Autodesk Inventor part; units mm, degrees
ref_plane "YZ Plane" through (0, 0, 0) normal (1, 0, 0) x (0, 1, 0)
ref_plane "XZ Plane" through (0, 0, 0) normal (0, 1, 0) x (-1, 0, 0)
ref_plane "XY Plane" through (0, 0, 0) normal (0, 0, 1) x (1, 0, 0)
sketch "Sketch1" plane through (0, 0, 0) normal (0, 0, 1) x (1, 0, 0)
  point P0 (0, 0)
sketch "Sketch2" plane through (0, 0, 0) normal (0, 0, 1) x (1, 0, 0)
  circle A0 centre (0, 0) radius 10
  line L0 (2.4793, 73.9585) -> (2.4781, 9.6881)
  line L1 (-2.5359, 9.6731) -> (-2.5218, 9.6731)
  line L2 (-2.5218, 9.6768) -> (-2.5207, 73.9571)
  line L3 (-2.4922, 73.958) -> (2.4781, 9.6881) construction
  line L4 (2.4804, 74.3269) -> (-2.5218, 9.6731) construction
  line L5 (-2.5218, 9.6731) -> (-2.5218, 9.6723)
  line L6 (9.283, 2.5) -> (74.717, 2.5)
  line L7 (74.717, 2.5) -> (74.717, -2.5)
  line L8 (74.717, -2.5) -> (9.283, -2.5)
  line L9 (9.283, -2.5) -> (9.283, 2.5)
  line L10 (9.283, 2.5) -> (74.717, -2.5) construction
  line L11 (74.717, 2.5) -> (9.283, -2.5) construction
  line L12 (2.4778, -7.9438) -> (2.5, -7.9438)
  line L13 (2.5, -9.6825) -> (2.5, -73.9578)
  line L14 (2.5, -76.0562) -> (2.4766, -76.0562)
  line L15 (-2.5, -73.9578) -> (-2.5, -9.6825)
  line L16 (-2.5, -7.9438) -> (2.5, -76.0562) construction
  line L17 (2.5, -7.9438) -> (-2.5, -76.0562) construction
  line L18 (-73.9602, 2.427) -> (-9.701, 2.427)
  line L19 (-8.7479, -2.5) -> (-8.7479, -2.573)
  line L20 (-9.6633, -2.573) -> (-73.9553, -2.573)
  line L21 (-75.2519, -2.573) -> (-75.2519, -2.5)
  line L22 (-75.2519, 2.427) -> (-8.7479, -2.573) construction
  line L23 (-8.7479, 2.427) -> (-75.2519, -2.573) construction
  line L24 (50.5283, 54.0638) -> (5.0788, 8.6143)
  line L25 (-1.7678, 1.7678) -> (1.7678, -1.7678)
  line L26 (8.6143, 5.0788) -> (54.0638, 50.5283)
  line L27 (53.4417, 51.1858) -> (5.5504, 8.3182) construction
  line L28 (39.6303, -7.8699) -> (34.6303, 82.4585) construction
  line L29 (-54.0638, -50.5283) -> (-8.6143, -5.0788)
  line L30 (-1.7678, 1.7678) -> (1.7678, -1.7678)
  line L31 (-5.0788, -8.6143) -> (-50.5283, -54.0638)
  line L32 (-51.9756, -52.6739) -> (-8.4008, -5.4246) construction
  line L33 (-52.6739, -51.9756) -> (-5.4246, -8.4008) construction
  arc A1 (73.9597, 2.4421) -> (53.4417, 51.1858) centre (0, 0) ccw
  arc A2 (50.5283, 54.0638) -> (2.452, 73.9594) centre (0, 0) ccw
  arc A3 (-73.9586, -2.4757) -> (-54.0638, -50.5283) centre (0, 0) ccw
  arc A4 (-50.5283, -54.0638) -> (-2.3463, -73.9628) centre (0, 0) ccw
  line L34 (-50.5283, 54.0638) -> (-5.0788, 8.6143)
  line L35 (1.7678, 1.7678) -> (0, 0)
  line L36 (-8.6143, 5.0788) -> (-54.0638, 50.5283)
  line L37 (-84.1138, 80.5783) -> (-5.4456, 8.3872) construction
  line L38 (-80.5783, 84.1138) -> (-1.7678, -1.7678) construction
  arc A5 (-2.4922, 73.958) -> (-50.5283, 54.0638) centre (0, 0) ccw
  arc A6 (-54.0638, 50.5283) -> (-73.9633, 2.3301) centre (0, 0) ccw
  line L39 (5.0788, -8.6143) -> (50.5283, -54.0638)
  line L40 (79.0888, -76.0562) -> (79.3403, -75.8047)
  line L41 (54.0638, -50.5283) -> (8.6143, -5.0788)
  line L42 (1.7678, 1.7678) -> (75.8047, -79.3403) construction
  line L43 (-1.7678, -1.7678) -> (79.3403, -75.8047) construction
  arc A7 (2.3463, -73.9628) -> (50.5283, -54.0638) centre (0, 0) ccw
  arc A8 (54.0638, -50.5283) -> (73.9597, -2.4421) centre (0, 0) ccw
  point P0 (-0.0207, 42)
  point P1 (-0.0207, 74.3122)
  point P2 (42, 0)
  point P3 (0, -42)
  point P4 (-41.9999, -0.073)
  point P5 (37.1303, 37.2943)
  point P6 (-43.6953, -43.6953)
  point P7 (-41.173, 41.173)
  point P8 (38.7862, -38.7862)
  point P9 (73.9578, -2.5)
  point P10 (73.9578, 2.5)
  dimension "d1" = 20
  dimension "d3" = 5
  dimension "d4" = 65.434
  dimension "d5" = 5
  dimension "d6" = 5
  dimension "d7" = 66.504
  dimension "d8" = 5
  dimension "d9" = 5
  dimension "d10" = 5
  dimension "d11" = 5
  dimension "d12" = 5
extrude "Extrusion1" add sketch "Sketch2" along normal blind 90 contours A0 L6 L9 L8 | L26 A1 L6 A0 | A0 L0 A2 L24 | A0 L34 A5 L2 | L8 A8 L41 A0 | L39 A7 L13 A0 | A0 L18 A6 L36 | L15 A4 L31 A0 | A0 L29 A3 L20 picked at (2.8651, 0.2554)
sketch "Sketch3" plane through (0, 0, 0) normal (0, 0, -1) x (-1, 0, 0)
  circle A0 centre (0, 0) radius 74
extrude "Extrusion2" add sketch "Sketch3" along normal blind 5
sketch "Sketch4" plane through (0, 0, 90) normal (0, 0, 1) x (1, 0, 0)
  circle A0 centre (0, 0) radius 73.9097
extrude "Extrusion3" add sketch "Sketch4" along normal blind 5
sketch "Sketch5" plane through (0, 0, 95) normal (0, 0, 1) x (1, 0, 0)
  circle A0 centre (0, 0) radius 2.5
  dimension "d19" = 5
extrude "Extrusion4" cut sketch "Sketch5" against normal through all
Model file for the job. Use its own axes, mm. A direction names the side the tool comes from. Give positions to 0.01 mm unless a question says otherwise; leave off trailing zeros. Order: outer loops, then holes, each group sorted by start corner. A loop starts at its lowest first (then second) coordinate and runs counter-clockwise, first axis right, second up. Notation, with made-up numbers: (71, 88.5) - (83, 88.5) arc R28 ccw to (83, 125.5) - close; hole circle Ø2 at (-31.5, 4). An arc over 180 degrees is marked (long way). Write item = value, one per line. Start each with the question number.
1. Cut at B-B, the plane x = 21.5. List the corners of the cut face in (y, z).
2. Cut at A-A, the plane x = 0. List the corners of the cut face in (y, z), and give its area (3 significant figures).
3. Two-plate mould, pull along Y, no slides. Class faces 4 (the cylindrical face through (16.04, 72.24, -2.46)), 5 (the flat face through (0, 42, 90)), 6 (the flat face through (9.283, 0, 44)): pulls with the +Y half, pulls with the -Y half, needs draft (parallel to the pull), parting line crosses it, or undercut.
4. Drop flat-ended pins along their axis: P1, Ø19.5, axis at x = 27, z = 23.5, coming from the +Y side; P2, Ø8, axis at y = -18.5, z = 72, coming from the +X side; P3, Ø1, axis at y = 3.5, z = 14, coming from the -X side. Give the stop position or say it passes through.
5. Cut at D-D, the plane y = 25.5. List the corners of the cut face in (x, z).
6. Which spindle directions (+Z, -Z, +X, -X, +Y, -Y) get a long thin tool onto all of the face, cutting with end or side? Do faces 1 (the flat face through (-41, 0, 0)), 2 (the flat face through (30, 30, 0)), 3 (the cylindrical face through (-0.54, -2.44, 45.7)). Say none if no direction does.
7. Probe line 1 along Y through (x, z) = (0, 15.5); line 2 along Y through (x, z) = (6, 6.5); line 3 along X through (y, z) = (-31, 49). List the from-to ranges inside material, lowest first.
Taken from the geometry:
q1.outline = (-70.81, -5) - (70.81, -5) - (70.81, 90) - (70.71, 90) - (70.71, 95) - (-70.71, 95) - (-70.71, 90) - (-70.81, 90) - close; hole (-25.04, 0) - (-17.96, 0) - (-17.96, 90) - (-25.04, 90) - close; hole (-2.5, 0) - (2.5, 0) - (2.5, 90) - (-2.5, 90) - close; hole (17.96, 0) - (25.04, 0) - (25.04, 90) - (17.96, 90) - close
q2.outline = (-74, -5) - (-2.5, -5) - (-2.5, 95) - (-73.91, 95) - (-73.91, 90) - (-10, 90) - (-10, 0) - (-74, 0) - close; (2.5, -5) - (74, -5) - (74, 0) - (10, 0) - (10, 90) - (73.91, 90) - (73.91, 95) - (2.5, 95) - close
q2.area = 2,780 mm²
q3.face_4 = parting line crosses it
q3.face_5 = needs draft
q3.face_6 = undercut
q4.P1 = 71.96
q4.P2 = 72.57
q4.P3 = -73.94
q5.outline = (-69.47, -5) - (69.47, -5) - (69.47, 90) - (69.37, 90) - (69.37, 95) - (-69.37, 95) - (-69.37, 90) - (-69.47, 90) - close; hole (-29.04, 0) - (-21.96, 0) - (-21.96, 90) - (-29.04, 90) - close; hole (-2.52, 0) - (2.48, 0) - (2.48, 90) - (-2.52, 90) - close; hole (21.96, 0) - (29.04, 0) - (29.04, 90) - (21.96, 90) - close
q6.face_1 = -X
q6.face_2 = none
q6.face_3 = +Z, -Z
q7.line_1 = -10 to -2.5, 2.5 to 10
q7.line_2 = -73.76 to -9.54, -8 to 8, 9.54 to 73.76
q7.line_3 = -67.19 to -34.54, -27.46 to -2.5, 2.5 to 27.46, 34.54 to 67.19
